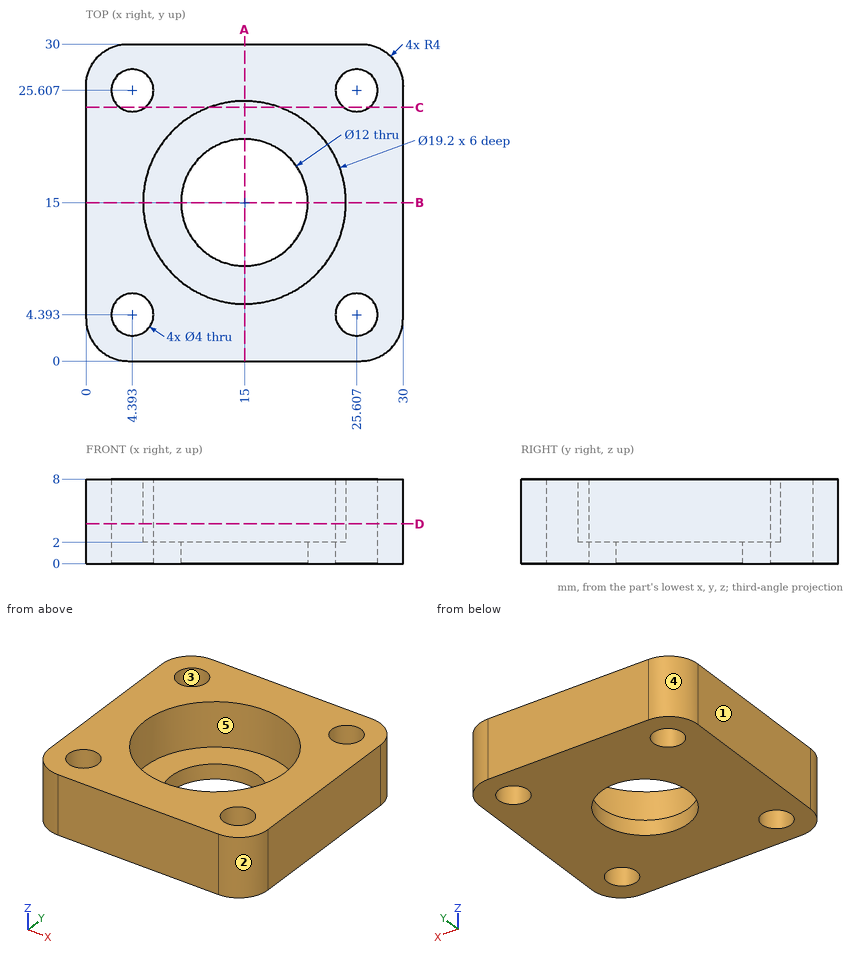
Verification items for this drawing (mm, ordinates from the low corner). A direction names the side the tool comes from. Give positions to 0.01 mm unless a question says otherwise; leave off trailing zeros. Write each loop counter-clockwise with the first axis right and the second up, starting at its lowest first coordinate (ties: lowest second). Pieces come first, ordered by that corner, then holes. Notation, with made-up numbers: (-27, 83.25) - (-19, 83.25) arc R18 cw to (-19, 92.25) - close; hole circle Ø10 at (61.5, -1.5). An arc over 180 degrees is marked (long way). Answer as a JSON object with one key per item and string values. Group by question number.
1) Access from +Z, -Z, +X, -X, +Y, -Y to the whole of each face (thin tool, end or side, straight path). Record for the marked faces 4 and 5.
2) Sectioned sample at A-A (x = 15). Record the cut outline in (y, z), then the cut area to 3 significant figures.
3) Thickness scan on probe 1 along X at (y, z) = (7.5, 6.75) (1 decimal); probe 2 along Y at (x, z) = (10.75, 6); probe 3 along Y at (x, z) = (15, 5.3). Record the ranges inside material, lowest first. Write a range as from..to.
4) Sectioned sample at C-C (y = 24). Record the cut outline in (x, z) (1 decimal), then the cut area to 3 significant figures.
5) Depth check by flat-ended pin: P1, Ø2.5, axis at x = 4.39, y = 4.39, coming from the -Z side. Enter the tip coordinate at first touch or a pass-through.
6) Sectioned sample at D-D (z = 3.75). Record the cut outline in (x, y).
7) Release check for a two-part mould opening along Y. For the marked faces 1, 2 and 3 record: pulls with the +Y half, pulls with the -Y half, needs draft (parallel to the pull), parting line crosses it, or undercut.
Geometry results:
{
 "1": {"face 4": "+Z, -Z, -X, +Y", "face 5": "+Z"},
 "2": {"outline": "(0, 0) - (9, 0) - (9, 2) - (5.4, 2) - (5.4, 8) - (0, 8) - close; (21, 0) - (30, 0) - (30, 8) - (24.6, 8) - (24.6, 2) - (21, 2) - close", "area": "101 mm^2"},
 "3": {"probe 1": "x = 0..9, 21..30", "probe 2": "y = 0..6.39, 23.61..30", "probe 3": "y = 0..5.4, 24.6..30"},
 "4": {"outline": "(0, 0) - (3.2, 0) - (3.2, 8) - (0, 8) - close; (5.6, 0) - (24.4, 0) - (24.4, 8) - (18.3, 8) - (18.3, 2) - (11.7, 2) - (11.7, 8) - (5.6, 8) - close; (26.8, 0) - (30, 0) - (30, 8) - (26.8, 8) - close", "area": "162 mm^2"},
 "5": {"P1": "passes through"},
 "6": {"outline": "(0, 4) arc R4 ccw to (4, 0) - (26, 0) arc R4 ccw to (30, 4) - (30, 26) arc R4 ccw to (26, 30) - (4, 30) arc R4 ccw to (0, 26) - close; hole circle Ø4 at (4.39, 4.39); hole circle Ø4 at (4.39, 25.61); hole circle Ø19.2 at (15, 15); hole circle Ø4 at (25.61, 4.39); hole circle Ø4 at (25.61, 25.61)"},
 "7": {"face 1": "needs draft", "face 2": "pulls with the -Y half", "face 3": "undercut"}
}
